from build123d import *

# Parameters (mm, degrees)
SKETCH1_R           = 30
SKETCH1_R_2         = 24.5
BOSS_EXTRUDE1_DEPTH = 20
CHAMFER2_SIZE       = 2.31
CHAMFER2_SIZE2      = 7
FILLET1_R           = 1


with BuildPart() as part:
    # Sketch1 → Boss-Extrude1 (new, symmetric)
    with BuildSketch(Plane(origin=(0, 0, 0), x_dir=(1, 0, 0), z_dir=(0, 1, 0))):
        with Locations(Location((0, 0, 0), (0, 0, 270))):
            Circle(SKETCH1_R)
        with Locations(Location((0, 0, 0), (0, 0, 270))):
            Circle(SKETCH1_R_2, mode=Mode.SUBTRACT)
    extrude(amount=BOSS_EXTRUDE1_DEPTH, both=True)

    # Chamfer2
    chamfer2_edges = [part.edges().sort_by_distance(p)[0] for p in [
        (0, -20, -30),
    ]]
    chamfer2_side = [part.faces().sort_by_distance(p)[0] for p in [
        (0, -20, -29.151471863),
    ]]
    chamfer(chamfer2_edges, length=CHAMFER2_SIZE, length2=CHAMFER2_SIZE2, reference=chamfer2_side[0])

    # Fillet1
    fillet1_edges = [part.edges().sort_by_distance(p)[0] for p in [
        (0, -20, -27.69),
        (0, 20, -30),
    ]]
    fillet(fillet1_edges, radius=FILLET1_R)


solid = part.part
Geometry: final body of the model. Coordinates: model frame, mm. Give positions to 0.01 mm unless a question says otherwise; leave off trailing zeros. Order: outer loops, then holes, each group sorted by start corner. A loop starts at its lowest first (then second) coordinate and runs counter-clockwise, first axis right, second up. Notation, with made-up numbers: (33.5, 70) -> (59.5, 70) arc R29 ccw to (59.5, 93) -> close; hole circle Ø5 at (-34, 25). An arc over 180 degrees is marked (long way). Write each question's results on one line, items separated by ' | '.
1) Cut plane C-C (y = 2). Output: boundary loops of the cut face in (x, z).
Geometry says:
outline: circle Ø60 at (0, 0); hole circle Ø49 at (0, 0)
2) Draft query along Z for faces 1 (the face through (24, 20, -7)), 2 (the face through (-27.38, -18.92, -6.08)), 3 (the face through (7.36, -0.28, 23.37)). Return one class per face: released by +Z, released by -Z, zero draft, split by the parting line, or undercut.
Geometry says:
face 1: zero draft | face 2: split by the parting line | face 3: undercut
3) Cut plane A-A (x = 0). Output: boundary loops of the cut face in (y, z), and give its area (3 significant figures).
Geometry says:
outline: (-20, -26.97) arc R1 ccw to (-19.31, -27.92) -> (-13, -30) -> (19, -30) arc R1 ccw to (20, -29) -> (20, -24.5) -> (-20, -24.5) -> close; (-20, 24.5) -> (20, 24.5) -> (20, 29) arc R1 ccw to (19, 30) -> (-13, 30) -> (-19.31, 27.92) arc R1 ccw to (-20, 26.97) -> close | area: 423 mm²
4) Line query: line 1 along X through (y, z) = (5.5, 0.5); line 2 along X through (y, z) = (-10.5, -4); line 3 along Z through (x, y) = (-16, 15). Output: solid intervals per line, ascending.
Geometry says:
line 1: x = -30 to -24.49, 24.49 to 30 | line 2: x = -29.73 to -24.17, 24.17 to 29.73 | line 3: z = -25.38 to -18.55, 18.55 to 25.38
5) Cut plane B-B (z = 0). Output: boundary loops of the cut face in (x, y).
Geometry says:
outline: (-30, -13) -> (-27.92, -19.31) arc R1 ccw to (-26.97, -20) -> (-24.5, -20) -> (-24.5, 20) -> (-29, 20) arc R1 ccw to (-30, 19) -> close; (24.5, -20) -> (26.97, -20) arc R1 ccw to (27.92, -19.31) -> (30, -13) -> (30, 19) arc R1 ccw to (29, 20) -> (24.5, 20) -> close
6) First-contact query: pin 1 Ø6 at (x, y) = (14, -7) entering from +Z; pin 2 Ø1 at (y, z) = (10.5, 19) entering from -X; pin 3 Ø12 at (y, z) = (13.5, -19.5) entering from +X. Flat tips, straight axial feed; report the tip coordinate or a pass-through.
Geometry says:
pin 1: stops at z = 27.91 | pin 2: stops at x = -23.62 | pin 3: stops at x = 26.79
